Could you check a few things on this model? Use its own coordinates, in mm. Face numbers are marked on the shaded views. A direction names the side the tool comes from. Give positions to 0.01 mm unless a question says otherwise; leave off trailing zeros. Write each loop counter-clockwise with the first axis right and the second up, starting at its lowest first coordinate (ties: lowest second). Pieces come first, ordered by that corner, then holes. Notation, with made-up numbers: (-16, -30.75) - (-2, -30.75) arc R22 ccw to (-2, 4.25) - close; hole circle Ø1 at (70.5, 38.5). An arc over 180 degrees is marked (long way). Write item = value, one per line.
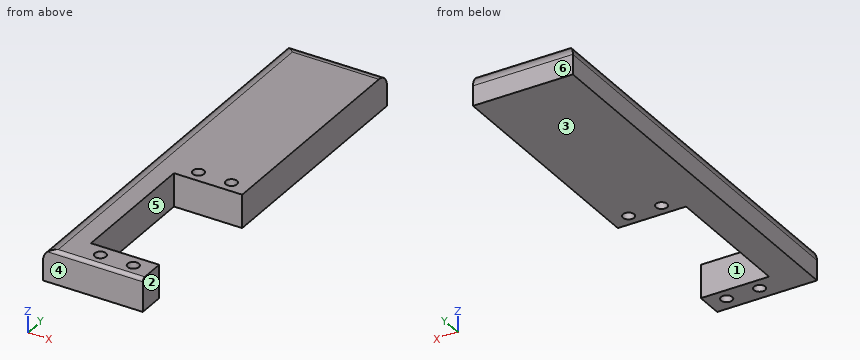
from build123d import *

# Parameters (mm, degrees)
SKETCH2_W           = 30
SKETCH2_H           = 120
BOSS_EXTRUDE1_DEPTH = 10
SKETCH3_R           = 1.7
SKETCH3_W           = 20.5
SKETCH3_H           = 40.8
CUT_EXTRUDE3_DEPTH  = 76.224148804
FILLET1_R           = 1
FILLET2_R           = 4


with BuildPart() as part:
    # Sketch2 → Boss-Extrude1 (new body)
    with BuildSketch(Plane.XY):
        with Locations((-15.991735537, -7.809917355)):
            Rectangle(SKETCH2_W, SKETCH2_H)
    extrude(amount=BOSS_EXTRUDE1_DEPTH)

    # Sketch3 → Cut-Extrude3 (cut, through all)
    with BuildSketch(Plane.XY):
        with Locations((-16.391735537, -63.486209282)):
            Circle(SKETCH3_R)
        with Locations((-6.491735537, -63.486209282)):
            Circle(SKETCH3_R)
        with Locations(Location((-6.491735537, -15.286209282, 0), (0, 0, 180))):
            Circle(SKETCH3_R)
        with Locations(Location((-16.391735537, -15.286209282, 0), (0, 0, 180))):
            Circle(SKETCH3_R)
        with Locations((-11.241735537, -39.386209282)):
            Rectangle(SKETCH3_W, SKETCH3_H)
    extrude(amount=CUT_EXTRUDE3_DEPTH, mode=Mode.SUBTRACT)

    # Fillet1
    fillet1_edges = [part.edges().sort_by_distance(p)[0] for p in [
        (-15.991735537, -67.809917355, 10),
    ]]
    fillet(fillet1_edges, radius=FILLET1_R)

    # Fillet2
    # the kernel refuses this fillet: 4 mm, written as the material it takes off along each edge
    with BuildSketch(Plane(origin=(-40.991735537, 52.190082645, 10), x_dir=(0, -1, 0), z_dir=(1, 0, 0))) as fillet2_piece_1:
        with BuildLine():
            CenterArc((FILLET2_R, FILLET2_R), FILLET2_R, 180, 90)
            Line((0, FILLET2_R), (0, 0))
            Line((0, 0), (FILLET2_R, 0))
        make_face()
    extrude(amount=50, mode=Mode.SUBTRACT)
    with BuildSketch(Plane(origin=(-30.991735537, -76.809917355, 10), x_dir=(0, 0, -1), z_dir=(0, 1, 0))) as fillet2_piece_2:
        with BuildLine():
            CenterArc((FILLET2_R, -FILLET2_R), FILLET2_R, 90, 90)
            Line((0, -FILLET2_R), (0, 0))
            Line((0, 0), (FILLET2_R, 0))
        make_face()
    extrude(amount=139, mode=Mode.SUBTRACT)


solid = part.part
1. If we section it at C-C, the plane x = -17: Please give me the cut outline in (y, z).
Filled sheet:
outline = (-67.81, 0) - (-65.07, 0) - (-65.07, 10) - (-66.81, 10) arc R1 ccw to (-67.81, 9) - close; (-61.9, 0) - (-59.79, 0) - (-59.79, 10) - (-61.9, 10) - close; (-18.99, 0) - (-16.87, 0) - (-16.87, 10) - (-18.99, 10) - close; (-13.7, 0) - (52.19, 0) - (52.19, 6) arc R4 ccw to (48.19, 10) - (-13.7, 10) - close
2. If we section it at B-B, the plane z = 2.25: Please give me the cut outline in (x, y), and give its area (3 significant figures).
Filled sheet:
outline = (-30.99, -67.81) - (-0.99, -67.81) - (-0.99, -59.79) - (-21.49, -59.79) - (-21.49, -18.99) - (-0.99, -18.99) - (-0.99, 52.19) - (-30.99, 52.19) - close; hole circle Ø3.4 at (-16.39, -63.49); hole circle Ø3.4 at (-16.39, -15.29); hole circle Ø3.4 at (-6.49, -63.49); hole circle Ø3.4 at (-6.49, -15.29)
area = 2,730 mm2
3. If we section it at D-D, the plane z = 7.5: Please give me the cut outline in (x, y).
Filled sheet:
outline = (-30.7, -67.81) - (-0.99, -67.81) - (-0.99, -59.79) - (-21.49, -59.79) - (-21.49, -18.99) - (-0.99, -18.99) - (-0.99, 51.9) - (-30.7, 51.9) - close; hole circle Ø3.4 at (-16.39, -63.49); hole circle Ø3.4 at (-16.39, -15.29); hole circle Ø3.4 at (-6.49, -63.49); hole circle Ø3.4 at (-6.49, -15.29)
4. Which directions (+Z, -Z, +X, -X, +Y, -Y) give clear straight access to the entire face, cutting with the end or side of a thin tool? Please do the marked faces 1 and 2.
Filled sheet:
face_1 = +Z, -Z, +X
face_2 = +Z, -Z, +X, +Y, -Y
5. Thinking about a two-plate mould opening in Y: for the marked faces 3, 4, 5 and 6, which applies, pulls with the +Y half, pulls with the -Y half, needs draft (parallel to the pull), parting line crosses it, or undercut?
Filled sheet:
face_3 = needs draft
face_4 = pulls with the -Y half
face_5 = undercut
face_6 = pulls with the +Y half
6. For pin 1 (4.5 mm diameter, centred on x = -6.49, y = -15.29, fed in from -Z), with a flat end and sliding along its axis, tell me the tip position at first contact or that it passes through.
Filled sheet:
pin_1 = 0
7. I need wall thicknesses on line 1 (Y direction, x = -6.5, z = 2); line 2 (Y direction, x = -19.5, z = 2.25); line 3 (Y direction, x = -17.5, z = 7.75). Which ranges of each line are inside material? Lowest first, please.
Filled sheet:
line_1 = -67.81 to -65.19, -61.79 to -59.79, -18.99 to -16.99, -13.59 to 52.19
line_2 = -67.81 to -59.79, -18.99 to 52.19
line_3 = -67.81 to -64.78, -62.2 to -59.79, -18.99 to -16.58, -14 to 51.79
8. If we section it at A-A, the plane y = -20: Please give me the cut outline in (x, z).
Filled sheet:
outline = (-30.99, 0) - (-21.49, 0) - (-21.49, 10) - (-26.99, 10) arc R4 ccw to (-30.99, 6) - close
